from build123d import *
from build123d.topology import SkipClean

# Parameters (mm, degrees)
SKETCH1_W                 = 44.45
SKETCH1_H                 = 44.45
SKETCH1_R                 = 2.38125
BOSS_EXTRUDE1_DEPTH       = 3.937
BOSS_EXTRUDE2_START       = 8.255
SKETCH3_W                 = 44.45
SKETCH3_H                 = 44.45
SKETCH3_R                 = 2.38125
BOSS_EXTRUDE2_DEPTH       = 8.255
F_2_56_TAPPED_HOLE1_D     = 1.778
F_2_56_TAPPED_HOLE1_DEPTH = 6.35
F_2_56_TAPPED_HOLE1_TIP   = 0.53416509


with BuildPart() as part:
    # Sketch1 → Boss-Extrude1 (new body)
    with BuildSketch(Plane(origin=(0, 0, 0), x_dir=(1, 0, 0), z_dir=(0, 1, 0))):
        Rectangle(SKETCH1_W, SKETCH1_H)
        with Locations(Location((0, 0, 0), (0, 0, 270))):
            Circle(SKETCH1_R, mode=Mode.SUBTRACT)
    extrude(amount=BOSS_EXTRUDE1_DEPTH)

    # Sketch3 → Boss-Extrude2 (add)
    with SkipClean():  # the faces are left unmerged after this step: merging them gives an invalid solid
        with BuildSketch(Plane.XZ.offset(BOSS_EXTRUDE2_START)):
            Rectangle(SKETCH3_W, SKETCH3_H)
            with Locations(Location((0, 0, 0), (0, 0, 270))):
                Circle(SKETCH3_R, mode=Mode.SUBTRACT)
        extrude(amount=-BOSS_EXTRUDE2_DEPTH)

    # #2-56 Tapped Hole1
    with Locations(Plane(origin=(0, 3.937, 0), x_dir=(1, 0, 0), z_dir=(0, 1, 0))):
        with Locations((15.947857811, -9.2075), (-15.947857811, -9.2075), (0, 18.415)):
            Hole(F_2_56_TAPPED_HOLE1_D / 2, depth=F_2_56_TAPPED_HOLE1_DEPTH)
            with Locations((0, 0, -(F_2_56_TAPPED_HOLE1_DEPTH + F_2_56_TAPPED_HOLE1_TIP / 2))):  # 118° drill point
                Cone(0, F_2_56_TAPPED_HOLE1_D / 2, F_2_56_TAPPED_HOLE1_TIP, mode=Mode.SUBTRACT)


solid = part.part
Model file for the job. Use its own axes, mm. A direction names the side the tool comes from. Coordinates: 2 decimals unless noted, no trailing zeros. Order: outer loops, then holes, each group sorted by start corner. A loop starts at its lowest first (then second) coordinate and runs counter-clockwise, first axis right, second up. Notation, with made-up numbers: (75, -13) -> (118, -13) arc R29 cw to (118, 16) -> close; hole circle Ø9 at (38.5, 31). An arc over 180 degrees is marked (long way). Return JSON: item names as keys, results as strings. Group by question number.
Item 1: Flat gauge pin, fed straight in: P1, Ø1.4, axis at x = 15.95, z = 9.21, coming from the +Y side. Where does the tip first touch, or does it go through?
Item 2: Pull direction Z, two halves, no side cores. Call faces 1 (the flat face through (0, -2, -22.225)), 2 (the conical face through (0.083, -2.854, -18.545)), 3 (the flat face through (0, -2, 22.225)), 4 (the flat face through (0, 3.937, -5)): pulls with the +Z half, pulls with the -Z half, needs draft (parallel to the pull), parting line crosses it, or undercut.
Item 3: Tool access for faces 5 (the flat face through (0, -8.255, 5)), 6 (the cylindrical face through (0.655, 0.718, -19.016)): list every direction of +Z, -Z, +X, -X, +Y, -Y with a clear straight run to the whole face (end or side of a thin tool).
Item 4: Saw through at A-A on z = 0. Write the cut outline in (x, y) (3 decimals).
Item 5: Wall check: line 1 along Z through (x, y) = (0, 1.25) (3 decimals); line 2 along X through (y, z) = (-4.75, 0) (3 decimals); line 3 along X through (y, z) = (0, -1.5) (3 decimals). Give the ranges that are in metal, low to high. Write a range as [from, to].
Values found:
{
 "1": {"P1": "stops at y = -2.52"},
 "2": {"face 1": "pulls with the -Z half", "face 2": "undercut", "face 3": "pulls with the +Z half", "face 4": "needs draft"},
 "3": {"face 5": "+Z, -Z, +X, -X, -Y", "face 6": "+Y"},
 "4": {"outline": "(-22.225, -8.255) -> (-2.381, -8.255) -> (-2.381, 3.937) -> (-22.225, 3.937) -> close; (2.381, -8.255) -> (22.225, -8.255) -> (22.225, 3.937) -> (2.381, 3.937) -> close"},
 "5": {"line 1": "z = [-22.225, -19.304], [-17.526, -2.381], [2.381, 22.225]", "line 2": "x = [-22.225, -2.381], [2.381, 22.225]", "line 3": "x = [-22.225, -1.849], [1.849, 22.225]"}
}
